Geometry: final body of the model. Coordinates: model frame, mm. Face numbers are marked on the shaded views. Round coordinates to 2 decimals unless told otherwise and drop trailing zeros. Write each loop counter-clockwise with the first axis right and the second up, starting at its lowest first coordinate (ties: lowest second). Pieces come first, ordered by that corner, then holes. Notation, with made-up numbers: (48, 88) -> (87, 88) arc R32 ccw to (87, 120) -> close; hole circle Ø10 at (19, 46). An arc over 180 degrees is marked (long way). Use one line per item in the form item = value. Start each with the question number.
1. Cut plane A-A, the plane z = 10.25. Return the cut outline in (x, y) (3 decimals).
2. Cut plane D-D, the plane z = 6. Return the cut outline in (x, y) (3 decimals).
3. Pin query (flat end, axial travel): pin 1 Ø3.5 at (y, z) = (-9.91, 9.12) entering from -X; pin 2 Ø5.5 at (y, z) = (11.5, 8.5) entering from +X; pin 3 Ø4.5 at (y, z) = (-9.91, 9.12) entering from +X (3 decimals); pin 4 Ø2.5 at (y, z) = (4.75, 3.18) entering from -X. Return the tip coordinate at first contact, or that it passes through.
4. Cut plane B-B, the plane y = 5. Return the cut outline in (x, z) (3 decimals), plus the area to 3 significant figures.
5. Line query: L1, parallel to Y at x = 5.5, z = 9.25; L2, parallel to Y at x = 7.25, z = 3.25; L3, parallel to X at y = 6, z = 5.25. Output: solid intervals per line, ascending.
6. Draft query along Z for the marked faces 1, 2, 3 and 4. Return one class per face: pulls with the +Z half, pulls with the -Z half, needs draft (parallel to the pull), parting line crosses it, or undercut.
7. Cut plane C-C, the plane x = 5.5. Return the cut outline in (y, z) (3 decimals).
```python
from build123d import *

# Parameters (mm, degrees)
F0_W     = 32.512
F0_H     = 21.59
F1_DEPTH = 12.7
F2_R     = 1.016
F2_R_2   = 1.905
F3_DEPTH = 12.701
F5_DEPTH = 1.651
F6_R     = 3.556
F7_DEPTH = 9.525


with BuildPart() as f1:
    # F0 (on Right) → F1 (new body)
    with BuildSketch(Plane.YZ):
        with Locations((0, 7.62)):
            Rectangle(F0_W, F0_H)
    extrude(amount=F1_DEPTH)

    # F2 (on face) → F3 (cut, through all)
    with BuildSketch(Plane(origin=(0, 0, 0), x_dir=(0, -1, 0), z_dir=(-1, 0, 0))):
        with Locations((4.7498, 3.175)):
            Circle(F2_R)
        with Locations((-4.7498, 3.175)):
            Circle(F2_R)
        with Locations((-9.906, 9.124435)):
            Circle(F2_R_2)
        with Locations((9.906, 9.124435)):
            Circle(F2_R_2)
    extrude(amount=-F3_DEPTH, mode=Mode.SUBTRACT)

    # F4 (on face) → F5 (cut)
    with BuildSketch(Plane(origin=(0, 0, 0), x_dir=(0, -1, 0), z_dir=(-1, 0, 0))):
        Polygon((-1.96794, 3.332093), (-3.494916, 5.662708), (-6.276777, 5.505615), (-7.53166, 3.017907), (-6.004684, 0.687292), (-3.222823, 0.844385), align=None)
        Polygon((6.142946, 5.588), (3.356654, 5.588), (1.963508, 3.175), (3.356654, 0.762), (6.142946, 0.762), (7.536092, 3.175), align=None)
    extrude(amount=-F5_DEPTH, mode=Mode.SUBTRACT)

    # F6 (on face) → F7 (cut)
    with BuildSketch(Plane.YZ.offset(12.7)):
        with Locations((9.906, 9.124435)):
            Circle(F6_R)
        with Locations((-9.906, 9.124435)):
            Circle(F6_R)
    extrude(amount=-F7_DEPTH, mode=Mode.SUBTRACT)


solid = f1.part
```
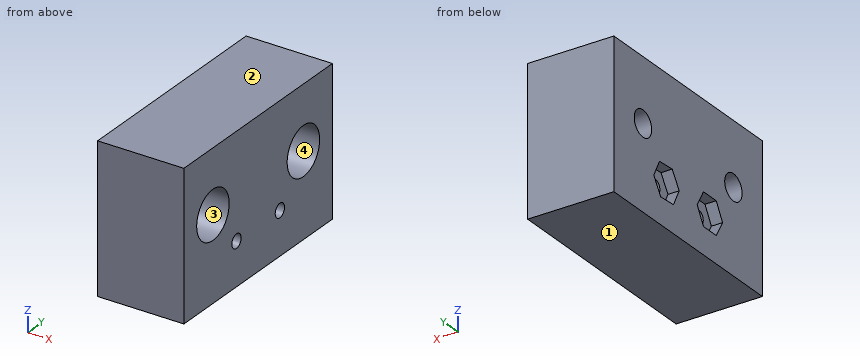
Outcome:
q1.outline = (0, -16.256) -> (12.7, -16.256) -> (12.7, -13.279) -> (3.175, -13.279) -> (3.175, -11.443) -> (0, -11.443) -> close; (0, -8.369) -> (3.175, -8.369) -> (3.175, -6.533) -> (12.7, -6.533) -> (12.7, 6.533) -> (3.175, 6.533) -> (3.175, 8.369) -> (0, 8.369) -> close; (0, 11.443) -> (3.175, 11.443) -> (3.175, 13.279) -> (12.7, 13.279) -> (12.7, 16.256) -> (0, 16.256) -> close
q2.outline = (0, -16.256) -> (12.7, -16.256) -> (12.7, -11.604) -> (3.175, -11.604) -> (3.175, -8.208) -> (12.7, -8.208) -> (12.7, 8.208) -> (3.175, 8.208) -> (3.175, 11.604) -> (12.7, 11.604) -> (12.7, 16.256) -> (0, 16.256) -> close
q3.pin_1 = through
q3.pin_2 = 12.7
q3.pin_3 = 3.175
q3.pin_4 = 1.65
q4.outline = (0, -3.175) -> (12.7, -3.175) -> (12.7, 2.19) -> (1.651, 2.19) -> (1.651, 0.744) -> (0, 0.744) -> close; (0, 5.578) -> (1.651, 5.578) -> (1.651, 4.16) -> (12.7, 4.16) -> (12.7, 18.415) -> (0, 18.415) -> close
q4.area = 244 mm^2
q5.L1 = -16.26 to -13.46, -6.35 to 6.35, 13.46 to 16.26
q5.L2 = -16.26 to -5.76, -3.74 to 3.74, 5.76 to 16.26
q5.L3 = 1.65 to 12.7
q6.face_1 = pulls with the -Z half
q6.face_2 = pulls with the +Z half
q6.face_3 = undercut
q6.face_4 = undercut
q7.outline = (-16.256, -3.175) -> (16.256, -3.175) -> (16.256, 18.415) -> (-16.256, 18.415) -> close; hole circle Ø7.112 at (-9.906, 9.124); hole circle Ø2.032 at (-4.75, 3.175); hole circle Ø2.032 at (4.75, 3.175); hole circle Ø7.112 at (9.906, 9.124)
